Design review of the part built by this model. Coordinates are the model's own, in mm. Give positions to 0.01 mm unless a question says otherwise; leave off trailing zeros. Order: outer loops, then holes, each group sorted by start corner. A loop starts at its lowest first (then second) coordinate and runs counter-clockwise, first axis right, second up. Notation, with made-up numbers: (-17, 0.5) -> (-11, 0.5) arc R22 ccw to (-11, 8.5) -> close; hole circle Ø1 at (-5, 48). An arc over 180 degrees is marked (long way). One line per item, written item: value. Start each with the question number.
1) Consider section C-C (y = 37.5). State how many separate pieces and enclosed holes the cut face has, plus the area to 3 significant figures.
2) Consider section B-B (z = -18). State the section outline as (x, y) points, plus the area to 3 significant figures.
3) Consider section A-A (z = 56). State the section outline as (x, y) points.
4) Wall thickness on line 1 along X through (y, z) = (38, 17.5); line 2 along Z through (x, y) = (9.25, 28.5); line 3 along Z through (x, y) = (9.75, 17.5): over which ranges is each line inside the solid? List them lowest first. Write a range as from..to.
5) For pin 1 (1.8 mm diameter, centred on y = 44.5, z = -1, fed in from +X); pin 2 (2 mm diameter, centred on y = 19, z = -0.5, fed in from +X), all flat-tipped, find the tip position at first contact; note any pin that passes through.
from build123d import *

# Parameters (mm, degrees)
PAD_DEPTH    = 70
POCKET_DEPTH = 8
CHAMFER_SIZE = 2


with BuildPart() as part:
    # Sketch → Pad (new body, symmetric)
    with BuildSketch(Plane.XY):
        with BuildLine():
            Line((0, 0), (0, 40))
            Line((0, 40), (3.5, 40))
            Line((3.5, 40), (3.5, 7))
            Line((3.5, 7), (7, 7))
            Line((7, 7), (7, 40))
            ThreePointArc((7, 40), (5.974874, 42.474874), (3.5, 43.5))
            Line((3.5, 43.5), (0, 43.5))
            Line((0, 43.5), (0, 47))
            Line((10.5, 47), (0, 47))
            Line((10.5, 47), (10.5, 0))
            Line((10.5, 0), (0, 0))
        make_face()
    extrude(amount=PAD_DEPTH, both=True)

    # Sketch001 (on Face1 of Pad) → Pocket (cut)
    with BuildSketch(Plane.YZ.offset(10.5)):
        Polygon((0, 1), (40, 1), (0, 41), (0, 43.828427), (42.414214, 1.414214), (62.414214, 21.414214), (62.414214, -21.414214), (42.414214, -1.414214), (0, -43.828427), (0, -41), (40, -1), (0, -1), align=None)
    extrude(amount=-POCKET_DEPTH, mode=Mode.SUBTRACT)

    # Chamfer
    chamfer_edges = [part.edges().sort_by_distance(p)[0] for p in [
        (10.5, 20, 1),
        (10.5, 20, -1),
        (10.5, 20, -21),
        (10.5, 21.207107, -22.62132),
        (10.5, 20, 21),
        (10.5, 21.207107, 22.62132),
    ]]
    chamfer(chamfer_edges, length=CHAMFER_SIZE)


solid = part.part
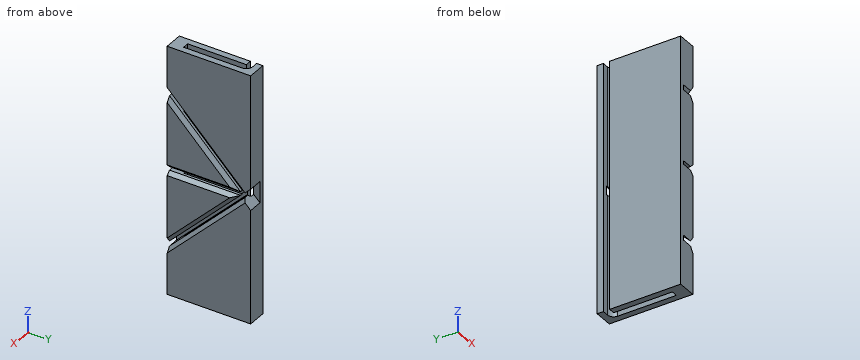
Checked values:
1. separate pieces: 5
1. enclosed holes: 0
1. area: 932 mm^2
2. outline: (0, 0) -> (10.5, 0) -> (10.5, 20.17) -> (8.5, 23) -> (7, 23) -> (7, 7) -> (3.5, 7) -> (3.5, 23) -> (2.5, 23) -> (2.5, 25.83) -> (3.5, 25.83) -> (3.5, 40) -> (0, 40) -> close; (0, 43.5) -> (3.5, 43.5) arc R3.5 cw to (7, 40) -> (7, 25.83) -> (8.5, 25.83) -> (10.5, 28.66) -> (10.5, 47) -> (0, 47) -> close
2. area: 338 mm^2
3. outline: (0, 0) -> (10.5, 0) -> (10.5, 47) -> (0, 47) -> (0, 43.5) -> (3.5, 43.5) arc R3.5 cw to (7, 40) -> (7, 7) -> (3.5, 7) -> (3.5, 40) -> (0, 40) -> close
4. line 1: x = 0..3.5, 7..10.5
4. line 2: z = -70..-16.39, -11.44..-1.75, 1.75..11.44, 16.39..70
4. line 3: z = -70..-28.1, -21.73..-2.25, 2.25..21.73, 28.1..70
5. pin 1: stops at x = 2.5
5. pin 2: stops at x = 9
